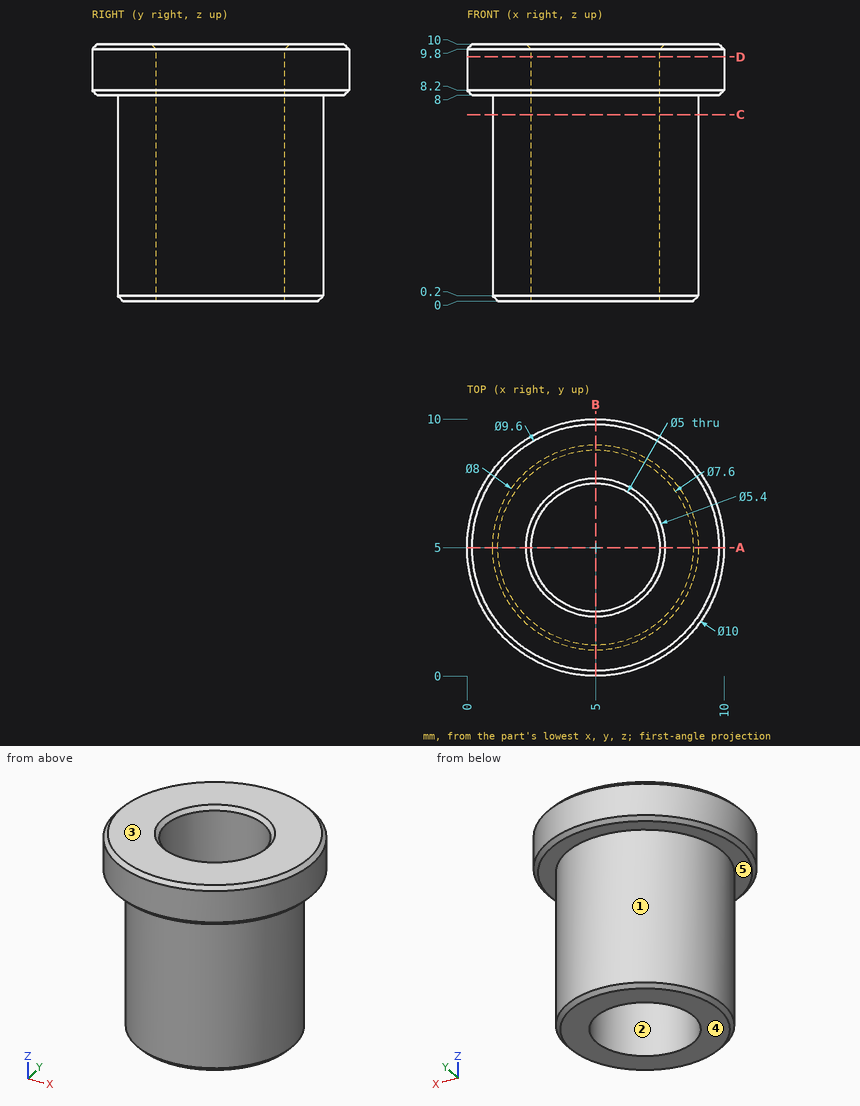
Input: dimensioned drawing with shaded views. Units: mm. Origin: part minimum x, y, z. A direction names the side the tool comes from. Coordinates: 2 decimals unless noted, no trailing zeros. Loops run counter-clockwise (first coordinate to the right, second up) from the corner with the lowest first, then second, coordinate; pieces in that order, holes last. Notation, with made-up numbers: M 71.5,5 L 113.5,5 A15 cw 113.5,26 Z; hole C -35.75,86.25 d4. An arc over 180 degrees is marked long. Use a Markdown table: item, result. Add a question column.
Q1. Draft query along X for the marked faces 1, 2 and 3. Return one class per face: pulls with the +X half, pulls with the -X half, needs draft (parallel to the pull), parting line crosses it, or undercut.
Q2. Material intervals for L1, parallel to Y at x = 5, z = 2.5; L2, parallel to Z at x = 9.25, y = 3.75; L3, parallel to X at y = 4.5, z = 3.5, sorted ascending.
Q3. Section query C-C, the plane z = 7.25. Return loops of the section in (x, y), and give its area (3 significant figures).
Q4. First-contact query: pin 1 (3 mm diameter, centred on x = 1, y = 3, fed in from -Z); pin 2 (4 mm diameter, centred on x = 5, y = 5, fed in from +Z); pin 3 (5 mm diameter, centred on x = 4.5, z = 4, fed in from +Y); pin 4 (1 mm diameter, centred on x = 8, z = 3.5, fed in from -Y). Flat tips, straight axial feed; report the tip coordinate or a pass-through.
Q5. Access query for the marked faces 4 and 5. Directions: +Z, -Z, +X, -X, +Y, -Y. A direction counts if a zero-diameter tool reaches every point of the face in a straight line with its end or side. Return the directions, or none.
Q6. Section query D-D, the plane z = 9.5. Return loops of the section in (x, y).
Q7. Section query A-A, the plane y = 5. Return loops of the section in (x, z), and give its area (3 significant figures).
Result:
| question | item | result |
|---|---|---|
| 1 | face 1 | parting line crosses it |
| 1 | face 2 | undercut |
| 1 | face 3 | needs draft |
| 2 | L1 | y = 1 to 2.5, 7.5 to 9 |
| 2 | L2 | z = 8 to 10 |
| 2 | L3 | x = 1.03 to 2.55, 7.45 to 8.97 |
| 3 | outline | C 5,5 d8; hole C 5,5 d5 |
| 3 | area | 30.6 mm2 |
| 4 | pin 1 | stops at z = 0 |
| 4 | pin 2 | passes through |
| 4 | pin 3 | stops at y = 9 |
| 4 | pin 4 | stops at y = 1.88 |
| 5 | face 4 | -Z, +X, -X, +Y, -Y |
| 5 | face 5 | -Z |
| 6 | outline | C 5,5 d10; hole C 5,5 d5 |
| 7 | outline | M 0,8.2 L 0.2,8 L 1,8 L 1,0.2 L 1.2,0 L 2.5,0 L 2.5,9.8 L 2.3,10 L 0.2,10 L 0,9.8 Z; M 7.5,0 L 8.8,0 L 9,0.2 L 9,8 L 9.8,8 L 10,8.2 L 10,9.8 L 9.8,10 L 7.7,10 L 7.5,9.8 Z |
| 7 | area | 33.8 mm2 |
